```python
from build123d import *

# Parameters (mm, degrees)
CHAMFER1_SIZE = 0.5


with BuildPart() as part:
    # Sketch1 → Revolve1 (revolve)
    with BuildSketch(Plane(origin=(0, 0, 0), x_dir=(1, 0, 0), z_dir=(0, 1, 0))):
        Polygon((-2.5, 0), (-2.5, 13), (-9, 13), (-9, 12), (-6, 12), (-6, 1), (-9, 1), (-9, 0), align=None)
    revolve(axis=Axis((0, 0, 0), (0, 0, -1)))

    # Chamfer1
    chamfer1_edges = [part.edges().sort_by_distance(p)[0] for p in [
        (2.5, 0, -13),
        (2.5, 0, 0),
        (9, 0, -1),
        (9, 0, -12),
    ]]
    chamfer(chamfer1_edges, length=CHAMFER1_SIZE)


solid = part.part
```
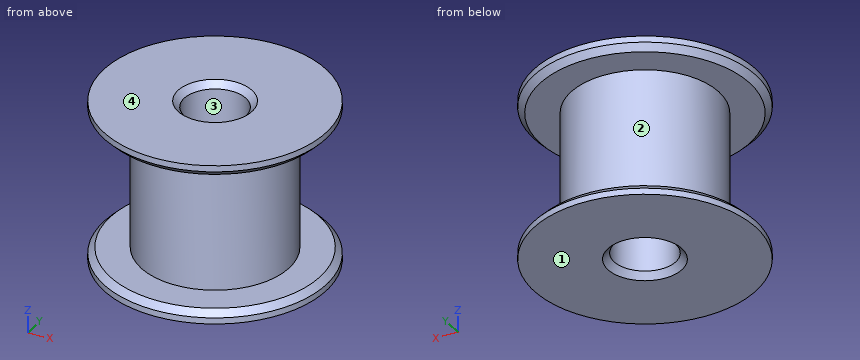
Model file for the job. Use its own axes, mm. Face numbers are marked on the shaded views. Give positions to 0.01 mm unless a question says otherwise; leave off trailing zeros. Loops run counter-clockwise (first coordinate to the right, second up) from the corner with the lowest first, then second, coordinate; pieces in that order, holes last. Notation, with made-up numbers: (38.5, -18.75) -> (54.5, -18.75) arc R27 cw to (54.5, 13.25) -> close; hole circle Ø3 at (-22.75, -30.5). An arc over 180 degrees is marked (long way). Use CSV: the item, a comma, the result in double quotes. Start each with the question number.
1) Flat gauge pins, fed straight in: pin 1 Ø4 at (y, z) = (7, -11.5) entering from +X; pin 2 Ø5 at (y, z) = (1.5, -6.5) entering from +X; pin 3 Ø4 at (x, z) = (6.5, -7) entering from +Y; pin 4 Ø4 at (x, y) = (0, 0) entering from +Z. Where does each tip first touch, or does it go through?
2) Wall check: line 1 (Y direction, x = 0, z = -8); line 2 (Z direction, x = 6, y = 3.5); line 3 (X direction, y = 0.5, z = -3.25). Give the ranges that are in metal, low to high.
3) Slice it at D-D on z = -0.75. Give the cut face in (x, y), plus the area to 3 significant figures.
4) Slice it at A-A on x = 0. Give the cut face in (y, z), plus the area to 3 significant figures.
5) Mould opens along Z. For the marked faces 1, 2, 3 and 4 say: released by +Z, released by -Z, zero draft, split by the parting line, or undercut.
6) Slice it at C-C on z = -11.75. Give the cut face in (x, y), plus the area to 3 significant figures.
Computed values:
1,pin 1,"stops at x = 7.3"
1,pin 2,"stops at x = 6"
1,pin 3,"stops at y = 3.97"
1,pin 4,"passes through"
2,line 1,"y = -6 to -2.5, 2.5 to 6"
2,line 2,"z = -13 to -12, -1 to 0"
2,line 3,"x = -5.98 to -2.45, 2.45 to 5.98"
3,outline,"circle Ø17.5 at (0, 0); hole circle Ø5 at (0, 0)"
3,area,"221 mm^2"
4,outline,"(-9, -13) -> (-3, -13) -> (-2.5, -12.5) -> (-2.5, -0.5) -> (-3, 0) -> (-9, 0) -> (-9, -0.5) -> (-8.5, -1) -> (-6, -1) -> (-6, -12) -> (-8.5, -12) -> (-9, -12.5) -> close; (2.5, -12.5) -> (3, -13) -> (9, -13) -> (9, -12.5) -> (8.5, -12) -> (6, -12) -> (6, -1) -> (8.5, -1) -> (9, -0.5) -> (9, 0) -> (3, 0) -> (2.5, -0.5) -> close"
4,area,"102 mm^2"
5,face 1,"released by -Z"
5,face 2,"undercut"
5,face 3,"zero draft"
5,face 4,"released by +Z"
6,outline,"circle Ø12 at (0, 0); hole circle Ø5 at (0, 0)"
6,area,"93.5 mm^2"
